```python
from build123d import *

# Parameters (mm, degrees)
F0_W     = 51.944476
F0_H     = 51.944479
F1_DEPTH = 7.62
F2_T     = -2.54
F5_DEPTH = 5.08


with BuildPart() as f1:
    # F0 (on Top) → F1 (new body)
    with BuildSketch(Plane.XY):
        with Locations((25.972238, -25.97224)):
            Rectangle(F0_W, F0_H)
    extrude(amount=F1_DEPTH)

    # F2
    f2_openings = [f1.faces().sort_by_distance(p)[0] for p in [
        (25.972238, -25.97224, 7.62),
    ]]
    offset(amount=F2_T, openings=f2_openings)

    # F3 (on face) → F5 (join)
    with BuildSketch(Plane.XY.offset(2.54)):
        Polygon((12.361643, -13.724343), (14.503031, -13.335001), (34.554198, -13.724343), (34.554198, -10.651178), (12.361643, -10.220256), align=None)
    extrude(amount=F5_DEPTH)


solid = f1.part
```
Read the model definition and answer for the solid it produces. Units are mm, in the model's axes. A direction names the side the tool comes from. Give positions to 0.01 mm unless a question says otherwise; leave off trailing zeros. Order: outer loops, then holes, each group sorted by start corner. A loop starts at its lowest first (then second) coordinate and runs counter-clockwise, first axis right, second up. Notation, with made-up numbers: (-11.75, 45.25) -> (42.25, 45.25) arc R25 cw to (42.25, 73.25) -> close; hole circle Ø1 at (15.5, 27.25). An arc over 180 degrees is marked (long way). One line per item, written item: value. Start each with the question number.
(1) The part is cut by section C-C (y = -12). Determine the outline of the cut face in (x, z), and give its area (3 significant figures).
(2) The part is cut by section A-A (z = 4.25). Determine the outline of the cut face in (x, y) (3 decimals), and give its area (3 significant figures).
(3) For a pull along Y with two mould halves and no side action, classify faces 1 (the flat face through (34.554, -12, 5)), 2 (the flat face through (26, 0, 4)), 3 (the flat face through (26, -51.944, 4)) as released by +Y, released by -Y, zero draft, split by the parting line, or undercut.
(4) A tool of negligible diameter and unlimited length cuts with its end or side. For faces 4 (the flat face through (23, -12, 7.62)), 5 (the flat face through (13.42, -13.53, 5.04)), from which of +Z, -Z, +X, -X, +Y, -Y can it reach the whole face along a straight path? Write none if from no direction.
(5) The part is cut by section D-D (y = -17.5). Determine the outline of the cut face in (x, z), and give its area (3 significant figures).
(6) Straight lines are drawn through the part: L1, parallel to Y at x = 48.5, z = 4.25; L2, parallel to X at y = -43, z = 7; L3, parallel to Y at x = 27.5, z = 5.25. For each, find the intervals that lie inside material, in ascending order.
(7) The part is cut by section B-B (x = 45.5). Determine the outline of the cut face in (y, z), and give its area (3 significant figures).
(8) Flat-ended cylindrical pins translate along their axes: P1, Ø4, axis at y = -16, z = 4, coming from the -X side; P2, Ø2, axis at x = 38, y = -25.5, coming from the +Z side. Find the tip coordinate at first contact, or state that the pin passes through.
Taken from the geometry:
1. outline: (0, 0) -> (51.94, 0) -> (51.94, 7.62) -> (49.4, 7.62) -> (49.4, 2.54) -> (34.55, 2.54) -> (34.55, 7.62) -> (12.36, 7.62) -> (12.36, 2.54) -> (2.54, 2.54) -> (2.54, 7.62) -> (0, 7.62) -> close
1. area: 270 mm^2
2. outline: (0, -51.944) -> (51.944, -51.944) -> (51.944, 0) -> (0, 0) -> close; (12.362, -13.724) -> (14.503, -13.335) -> (34.554, -13.724) -> (34.554, -10.651) -> (12.362, -10.22) -> close; hole (2.54, -49.404) -> (49.404, -49.404) -> (49.404, -2.54) -> (2.54, -2.54) -> close
2. area: 571 mm^2
3. face 1: undercut
3. face 2: released by +Y
3. face 3: released by -Y
4. face 4: +Z, +X, -X, +Y, -Y
4. face 5: +Z
5. outline: (0, 0) -> (51.94, 0) -> (51.94, 7.62) -> (49.4, 7.62) -> (49.4, 2.54) -> (2.54, 2.54) -> (2.54, 7.62) -> (0, 7.62) -> close
5. area: 158 mm^2
6. L1: -51.94 to -49.4, -2.54 to 0
6. L2: 0 to 2.54, 49.4 to 51.94
6. L3: -51.94 to -49.4, -13.59 to -10.51, -2.54 to 0
7. outline: (-51.94, 0) -> (0, 0) -> (0, 7.62) -> (-2.54, 7.62) -> (-2.54, 2.54) -> (-49.4, 2.54) -> (-49.4, 7.62) -> (-51.94, 7.62) -> close
7. area: 158 mm^2
8. P1: x = 0
8. P2: z = 2.54
